Autodesk Inventor part; units mm, degrees
ref_plane "Work Plane1" through (0, 8, 0) normal (0, -1, 0) x (1, 0, 0)
ref_plane "YZ Plane" through (0, 0, 0) normal (1, 0, 0) x (0, 1, 0)
ref_plane "XZ Plane" through (0, 0, 0) normal (0, 1, 0) x (-1, 0, 0)
sketch "Sketch1" plane through (0, 0, 0) normal (0, 1, 0) x (-1, 0, 0)
  circle A0 centre (0, 0) radius 10.875
  dimension "d0" = 21.75
extrude "Extrusion1" add sketch "Sketch1" along normal blind 43.6
sketch "Sketch2" plane through (0, 0, 0) normal (0, -1, 0) x (1, 0, 0)
  circle A0 centre (0, 0) radius 2
  dimension "d3" = 4
extrude "Extrusion2" cut sketch "Sketch2" against normal through all
sketch "Sketch3" plane through (0, 0, 0) normal (0, -1, 0) x (1, 0, 0)
  line L0 (-2, -6.1847) -> (-2, 6.1847)
  line L1 (2, 6.1847) -> (2, -6.1847)
  arc A0 (2, 6.1847) -> (-2, 6.1847) centre (0, 0) ccw
  arc A1 (-2, -6.1847) -> (2, -6.1847) centre (0, 0) ccw
  dimension "d26" = 6.5
  dimension "d27" = 4
  dimension "d28" = 2
extrude "Extrusion3" cut sketch "Sketch3" against normal blind 12
sketch "Sketch4" plane through (0, 12, 0) normal (0, -1, 0) x (1, 0, 0)
  line L0 (2, -7.1361) -> (-2, -7.1361) construction
  line L1 (-2, -7.1361) -> (-2, 7.9296) construction
  line L2 (-2, 7.9296) -> (2, 7.9296) construction
  line L3 (2, 7.9296) -> (2, -7.1361) construction
  line L4 (7.1801, -1.836) -> (5.1801, -5.3001) construction
  line L5 (5.1801, -5.3001) -> (-7.8673, 2.2328) construction
  line L6 (-7.8673, 2.2328) -> (-5.8673, 5.6969) construction
  line L7 (-5.8673, 5.6969) -> (7.1801, -1.836) construction
  arc A0 (-2, 6.1847) -> (-6.3561, 1.3603) centre (0, 0) ccw
  arc A1 (2, -6.1847) -> (6.3561, -1.3603) centre (0, 0) ccw
  line L8 (-2, 6.1847) -> (-2, 3.4641)
  line L9 (6.3561, -1.3603) -> (-2, 3.4641)
  line L10 (2, -6.1847) -> (2, -3.4641)
  line L11 (2, -3.4641) -> (-6.3561, 1.3603)
  dimension "d29" = 4
  dimension "d32" = 60
extrude "Extrusion4" cut sketch "Sketch4" along normal blind 4.5
ref_plane "Work Plane1" through (0, 8, 0) normal (0, -1, 0) x (1, 0, 0)
sketch "Sketch5" plane through (0, 8, 0) normal (0, -1, 0) x (1, 0, 0)
  line L0 (2, -9.381) -> (-2, -9.381) construction
  line L1 (-2, -9.381) -> (-2, 10.3615) construction
  line L2 (-2, 10.3615) -> (2, 10.3615) construction
  line L3 (2, 10.3615) -> (2, -9.381) construction
  line L4 (9.1242, -2.9584) -> (7.1242, -6.4225) construction
  line L5 (7.1242, -6.4225) -> (-9.9734, 3.4487) construction
  line L6 (-9.9734, 3.4487) -> (-7.9734, 6.9128) construction
  line L7 (-7.9734, 6.9128) -> (9.1242, -2.9584) construction
  line L8 (7.1242, 6.4225) -> (9.1242, 2.9584) construction
  line L9 (9.1242, 2.9584) -> (-7.9734, -6.9128) construction
  line L10 (-7.9734, -6.9128) -> (-9.9734, -3.4487) construction
  line L11 (-9.9734, -3.4487) -> (7.1242, 6.4225) construction
  line L12 (2, -3.4641) -> (4.3561, -4.8244)
  line L13 (2, 6.1847) -> (2, 1.1547)
  line L14 (0, 2.3094) -> (2, 1.1547)
  line L15 (2, 1.1547) -> (2, -3.4641)
  line L16 (-2, 3.4641) -> (-4.3561, 4.8244)
  line L17 (-2, -6.1847) -> (-2, -1.1547)
  line L18 (-2, 3.4641) -> (-2, -1.1547)
  line L19 (-2, -1.1547) -> (0, -2.3094)
  line L20 (-4.3561, -4.8244) -> (0, -2.3094)
  arc A0 (-4.3561, 4.8244) -> (-4.3561, -4.8244) centre (0, 0) ccw
  arc A1 (4.3561, -4.8244) -> (4.3561, 4.8244) centre (0, 0) ccw
  line L21 (0, 2.3094) -> (4.3561, 4.8244)
  dimension "d37" = 4
  dimension "d40" = 60
  dimension "d44" = 60
extrude "Extrusion5" cut sketch "Sketch5" along normal blind 4
sketch "Sketch6" plane through (0, 0, 0) normal (0, -1, 0) x (1, 0, 0)
  circle A0 centre (0, 0) radius 4.8
  dimension "d49" = 9.6
extrude "Extrusion6" cut sketch "Sketch6" against normal blind 27
sketch "Sketch7" plane through (0, 43.6, 0) normal (0, 1, 0) x (1, 0, 0)
  line L0 (0, 0) -> (8.3053, 8.3053) construction
  line L1 (0, 0) -> (11.7454, 0) construction
  point P0 (5.1265, 5.1265)
  point P1 (-5.1265, -5.1265)
  dimension "d68" = 45
  dimension "d69" = 14.5
  dimension "d70" = 7.25
hole "Hole1" at (-5.1265, 43.6, 5.1265) at (5.1265, 43.6, -5.1265) direction (0, -1, 0) diameter 1.567 depth 5 tip angle 118
properties part number "EncoderHandleSupport"
For this review, take the finished solid that the model builds, in its own axes (mm). A direction names the side the tool comes from. Round coordinates to 2 decimals unless told otherwise and drop trailing zeros. Write each loop counter-clockwise with the first axis right and the second up, starting at its lowest first coordinate (ties: lowest second). Pieces come first, ordered by that corner, then holes. Notation, with made-up numbers: (-8.75, 56.5) - (46.25, 56.5) arc R25 ccw to (46.25, 71.5) - close; hole circle Ø6 at (76.25, 55.5). An arc over 180 degrees is marked (long way). Answer as a JSON object with one key per item and string values.
1. To check wall thickness, follow line 1 along Z through (x, y) = (0, 21) (3 decimals); line 2 along Z through (x, y) = (0, 5.75) (3 decimals); line 3 along Y through (x, z) = (-2, -2). State the ranges of each line that lie inside material, in increasing order.
Response values:
{"line 1": "z = -10.875 to -4.8, 4.8 to 10.875", "line 2": "z = -10.875 to -6.5, 6.5 to 10.875", "line 3": "y = 27 to 43.6"}
2. We need section D-D on x = 3.25. Give the boundary of the cut face in (y, z), then the cut area to 3 significant figures.
Response values:
{"outline": "(0, -10.38) - (43.6, -10.38) - (43.6, 10.38) - (0, 10.38) - (0, 3.53) - (4, 3.53) - (4, 4.19) - (8, 4.19) - (8, 3.53) - (27, 3.53) - (27, -3.53) - (12, -3.53) - (12, -5.63) - (7.5, -5.63) - (7.5, -4.19) - (4, -4.19) - (4, -3.53) - (0, -3.53) - close", "area": "700 mm2"}
3. We need section C-C on z = -3.25. Give the boundary of the cut face in (x, y).
Response values:
{"outline": "(-10.38, 0) - (-3.53, 0) - (-3.53, 4) - (-5.63, 4) - (-5.63, 8) - (-3.53, 8) - (-3.53, 27) - (3.53, 27) - (3.53, 12) - (5.63, 12) - (5.63, 4) - (3.53, 4) - (3.53, 0) - (10.38, 0) - (10.38, 43.6) - (-10.38, 43.6) - close"}
4. Draft analysis for pull direction Z (two halves, no side actions). For faces 1 (the face through (-2.3, 0, -4.7)), 2 (the face through (-3.579, 6.028, -4.375)), state which applies: +Z half, -Z half, draft (parallel to the pull), parting line (faces both ways), or undercut.
Response values:
{"face 1": "draft", "face 2": "undercut"}
5. For pin 1 Ø2 at (y, z) = (4, 5.5) entering from +X; pin 2 Ø1.3 at (x, z) = (-5.13, 5.13) entering from +Y; pin 3 Ø0.9 at (y, z) = (6, 5) entering from -X, all flat-tipped, find the tip position at first contact; note any pin that passes through.
Response values:
{"pin 1": "stops at x = 9.9", "pin 2": "stops at y = 38.52", "pin 3": "stops at x = -9.88"}
6. We need section B-B on y = 31.5. Give the boundary of the cut face in (x, z) (3 decimals), then the cut area to 3 significant figures.
Response values:
{"outline": "circle Ø21.75 at (0, 0); hole circle Ø4 at (0, 0)", "area": "359 mm2"}
7. Tool access review of faces 3 (the face through (-5, 8, -2)), 4 (the face through (5.6, 41.06, -5.75)), 5 (the face through (1, 27, -2)): name each direction out of +Z, -Z, +X, -X, +Y, -Y from which nothing blocks a thin tool from reaching the whole face with its end or side.
Response values:
{"face 3": "none", "face 4": "+Y", "face 5": "-Y"}
8. We need section A-A on x = 0. Give the boundary of the cut face in (y, z) (3 decimals).
Response values:
{"outline": "(0, -10.875) - (43.6, -10.875) - (43.6, -2) - (27, -2) - (27, -4.8) - (12, -4.8) - (12, -6.5) - (0, -6.5) - close; (0, 6.5) - (12, 6.5) - (12, 4.8) - (27, 4.8) - (27, 2) - (43.6, 2) - (43.6, 10.875) - (0, 10.875) - close"}
